Can you work these out from the model? Positions are in its coordinate system, mm. Face numbers are marked on the shaded views. Coordinates: 2 decimals unless noted, no trailing zeros. Order: outer loops, then holes, each group sorted by start corner. A loop starts at its lowest first (then second) coordinate and runs counter-clockwise, first axis right, second up. Notation, with made-up numbers: M 43.25,45.25 L 71.25,45.25 A19 cw 71.25,61.25 Z; hole C 79,-8 d5. An arc over 180 degrees is marked long. Answer as a JSON object with one key per item and string values.
Autodesk Inventor part; units mm, degrees
ref_plane "YZ Plane" through (0, 0, 0) normal (1, 0, 0) x (0, 1, 0)
ref_plane "XZ Plane" through (0, 0, 0) normal (0, 1, 0) x (-1, 0, 0)
ref_plane "XY Plane" through (0, 0, 0) normal (0, 0, 1) x (1, 0, 0)
sketch "Sketch1" plane through (0, 0, 0) normal (0, 1, 0) x (-1, 0, 0)
  line L0 (3, 3) -> (-3, 3)
  line L1 (-3, 3) -> (-3, -3)
  line L2 (-3, -3) -> (3, -3)
  line L3 (3, -3) -> (3, 3)
  line L4 (3, 3) -> (-3, -3) construction
  line L5 (-3, 3) -> (3, -3) construction
  point P0 (0, 0)
  dimension "d0" = 6
  dimension "d1" = 6
extrude "Extrusion1" add sketch "Sketch1" along normal blind 12
sketch "Sketch2" plane through (0, 0, 0) normal (0, -1, 0) x (1, 0, 0)
  line L0 (-1.7, -1.7) -> (1.7, -1.7)
  line L1 (1.7, -1.7) -> (1.7, 1.7)
  line L2 (1.7, 1.7) -> (-1.7, 1.7)
  line L3 (-1.7, 1.7) -> (-1.7, -1.7)
  line L4 (-1.7, -1.7) -> (1.7, 1.7) construction
  line L5 (1.7, -1.7) -> (-1.7, 1.7) construction
  point P0 (0, 0)
  dimension "d4" = 3.4
  dimension "d5" = 3.4
extrude "Extrusion2" cut sketch "Sketch2" against normal blind 3.8
sketch "Sketch3" plane through (0, 0, 0) normal (0, 0, 1) x (1, 0, 0)
  line L0 (-1.65, 0.7481) -> (1.65, 0.7481)
  line L1 (1.25, 1.7481) -> (1.25, 0.7481)
  line L2 (-1.65, 1.7481) -> (1.65, 1.7481)
  line L3 (-1.25, 0.7481) -> (-1.25, 1.7481)
  line L4 (1.7, 0) -> (1.7, 3.8)
  line L5 (1.7, 1.6241) -> (1.6, 1.6241)
  line L6 (1.6, 1.6241) -> (1.6, 0.8418)
  line L7 (1.6, 0.8418) -> (1.7, 0.8418)
  line L8 (1.7, 0.8418) -> (1.7, 1.6241)
  point P0 (0, 0)
  dimension "d8" = 0.1
extrude "Extrusion3" add sketch "Sketch3" along normal mid plane 3.8 contours L7 L6 L5 L4
mirror "Mirror1" about plane through (0, 0, 0) normal (1, 0, 0) of "Extrusion3"
fillet "Fillet1" radius 0.1 2 edges at (-1.6, 0.8418, 0) (1.6, 0.8418, 0)
fillet "Fillet2" radius 1 8 edges at (-3, 6, 3) (3, 6, 3) (3, 6, -3) (-3, 6, -3) (0, 12, 3) (-3, 12, 0) (0, 12, -3) (3, 12, 0)
properties part number "Button"
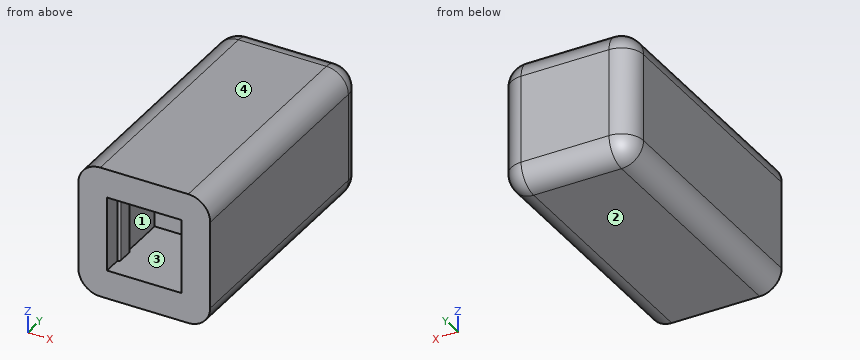
Item 1: I'm going to push flat-ended pins straight in: pin 1 (2 mm diameter, centred on x = 0, z = 0.5, fed in from -Y); pin 2 (1.5 mm diameter, centred on x = -2, z = -0.5, fed in from -Y). Where does each tip first touch, or does it pass through?
Answers follow:
{"pin 1": "stops at y = 3.8", "pin 2": "stops at y = 0"}
Item 2: I want a section at B-B, the plane y = 4.75. Write out the boundary of the cut face in (x, z), plus the area to 3 significant figures.
Answers follow:
{"outline": "M -3,-2 A1 ccw -2,-3 L 2,-3 A1 ccw 3,-2 L 3,2 A1 ccw 2,3 L -2,3 A1 ccw -3,2 Z", "area": "35.1 mm^2"}
Item 3: I want a section at D-D, the plane x = -1.4. Write out the boundary of the cut face in (y, z).
Answers follow:
{"outline": "M 0,-3 L 11,-3 A1 ccw 12,-2 L 12,2 A1 ccw 11,3 L 0,3 L 0,1.7 L 3.8,1.7 L 3.8,-1.7 L 0,-1.7 Z"}
Item 4: Please list where these lines run through material, in increasing order: line 1 (X direction, y = 1.75, z = -0.6); line 2 (Y direction, x = -0.2, z = 1.6).
Answers follow:
{"line 1": "x = -3 to -1.7, 1.7 to 3", "line 2": "y = 3.8 to 12"}
Item 5: If we mould it in two halves opening along Z, with no side actions, what happens to the marked faces 1, 2, 3 and 4? For each: pulls with the +Z half, pulls with the -Z half, needs draft (parallel to the pull), parting line crosses it, or undercut.
Answers follow:
{"face 1": "undercut", "face 2": "pulls with the -Z half", "face 3": "undercut", "face 4": "pulls with the +Z half"}
Item 6: I want a section at A-A, the plane y = 2.5. Write out the boundary of the cut face in (x, z), plus the area to 3 significant figures.
Answers follow:
{"outline": "M -3,-2 A1 ccw -2,-3 L 2,-3 A1 ccw 3,-2 L 3,2 A1 ccw 2,3 L -2,3 A1 ccw -3,2 Z; hole M -1.7,-1.7 L 1.7,-1.7 L 1.7,1.7 L -1.7,1.7 Z", "area": "23.6 mm^2"}
